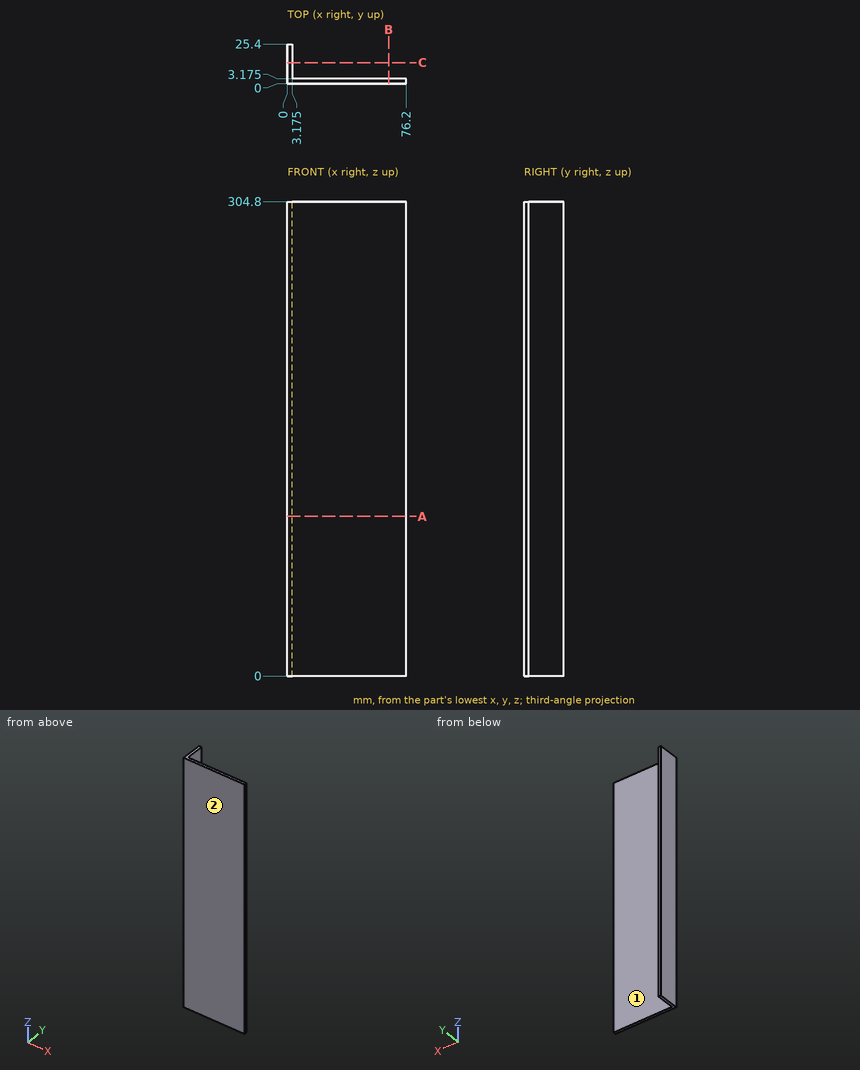
Could you check a few things on this drawing? It's one solid part, dimensions in mm from its lowest x, y, z. A direction names the side the tool comes from. Coordinates: 2 decimals unless noted, no trailing zeros. Write each loop counter-clockwise with the first axis right and the second up, starting at its lowest first coordinate (ties: lowest second). Pieces come first, ordered by that corner, then holes. Notation, with made-up numbers: (56.25, 9.5) - (72.25, 9.5) arc R22 cw to (72.25, 36.5) - close; hole circle Ø11 at (17.25, 19). An arc over 180 degrees is marked (long way). Write item = value, one per line.
1) Suppose I cut it at A-A on z = 102.5. Please give me the cut outline in (x, y) (3 decimals), plus the area to 4 significant figures.
Result set:
outline = (0, 0) - (76.2, 0) - (76.2, 3.175) - (3.175, 3.175) - (3.175, 25.4) - (0, 25.4) - close
area = 312.5 mm2
2) Suppose I cut it at B-B on x = 65. Please give me the cut outline in (y, z) (3 decimals).
Result set:
outline = (0, 0) - (3.175, 0) - (3.175, 304.8) - (0, 304.8) - close
3) Will these pins go through, and if not, where does the flat tip stop? pin 1 Ø22 at (x, z) = (56.5, 85) entering from +Y (3 decimals); pin 2 Ø8 at (y, z) = (15.5, 166) entering from +X (3 decimals).
Result set:
pin_1 = 3.175
pin_2 = 3.175
4) Please list where this line runs through material, in increasing order: line 1 (X direction, y = 11.25, z = 250) (3 decimals). Write a range as [from, to].
Result set:
line_1 = [0, 3.175]
5) For the marked faces 1 and 2, which set-ups out of +Z, -Z, +X, -X, +Y, -Y let a thin tool reach every point of the face, with its end or its side?
Result set:
face_1 = +Z, -Z, +X, +Y
face_2 = +Z, -Z, +X, -X, -Y
